```python
from build123d import *

# Parameters (mm, degrees)
SKETCH2_W           = 177.8
SKETCH2_H           = 58
BOSS_EXTRUDE2_DEPTH = 4
CUT_EXTRUDE1_REACH  = 6
SKETCH3_R           = 10.5


with BuildPart() as part:
    # Sketch2 → Boss-Extrude2 (new body)
    with BuildSketch(Plane.XY):
        with Locations((5.225854908, 0.185980872)):
            Rectangle(SKETCH2_W, SKETCH2_H)
    extrude(amount=BOSS_EXTRUDE2_DEPTH)

    # Sketch3 → Cut-Extrude1 (cut, up to next)
    with BuildSketch(Plane.XY.offset(4), mode=Mode.PRIVATE) as cut_extrude1_sk1:
        with Locations((5.225854908, 0.185980872)):
            Circle(SKETCH3_R)
    cut_extrude1_tool1 = extrude(cut_extrude1_sk1.sketch, amount=-CUT_EXTRUDE1_REACH, mode=Mode.PRIVATE) & part.part
    add(cut_extrude1_tool1.solids().sort_by_distance((5.225855, 0.185981, 4))[0], mode=Mode.SUBTRACT)


solid = part.part
```
CAD build for the part. Positions are in the model's coordinates, mm. Give positions to 0.01 mm unless a question says otherwise; leave off trailing zeros. Order: outer loops, then holes, each group sorted by start corner. A loop starts at its lowest first (then second) coordinate and runs counter-clockwise, first axis right, second up. Notation, with made-up numbers: M -17,81 L 11,81 A15 cw 11,110 Z; hole C 35,33 d1. An arc over 180 degrees is marked long. Put each result on its own line as item: value. Start each with the question number.
(1) Mould opens along Y. For faces 1 (the cylindrical face through (-3.11, -6.2, 2.03)), 2 (the flat face through (4, 29.186, 2)), 3 (the flat face through (4, -12, 0)), 4 (the flat face through (4, -28.814, 2)) say: +Y half, -Y half, draft (parallel to the pull), parting line (faces both ways), or undercut.
(2) Saw through at B-B, the plane x = -0.5. Write the cut outline in (y, z), then the cut area to 3 significant figures.
(3) Flat gauge pin, fed straight in: pin 1 Ø17 at (x, y) = (5.23, 0.19) entering from +Z. Where does the tip first touch, or does it go through?
(4) Saw through at A-A, the plane y = 4.5. Write the cut outline in (x, z).
(5) Saw through at C-C, the plane z = 1.8. Write the cut outline in (x, y), then the cut area to 3 significant figures.
(6) Drill centre lines: line 1 along Y through (x, z) = (4.5, 1.7); line 2 along X through (y, z) = (4.5, 3.55); line 3 along X through (y, z) = (-5, 1.1). Where is each one in solid material? Low to high.
Check result:
1. face 1: undercut
1. face 2: +Y half
1. face 3: draft
1. face 4: -Y half
2. outline: M -28.81,0 L -8.62,0 L -8.62,4 L -28.81,4 Z; M 8.99,0 L 29.19,0 L 29.19,4 L 8.99,4 Z
2. area: 162 mm2
3. pin 1: passes through
4. outline: M -83.67,0 L -4.35,0 L -4.35,4 L -83.67,4 Z; M 14.8,0 L 94.13,0 L 94.13,4 L 14.8,4 Z
5. outline: M -83.67,-28.81 L 94.13,-28.81 L 94.13,29.19 L -83.67,29.19 Z; hole C 5.23,0.19 d21
5. area: 9,970 mm2
6. line 1: y = -28.81 to -10.29, 10.66 to 29.19
6. line 2: x = -83.67 to -4.35, 14.8 to 94.13
6. line 3: x = -83.67 to -3.9, 14.36 to 94.13
